Could you check a few things on this drawing? It's one solid part, dimensions in mm from its lowest x, y, z. A direction names the side the tool comes from. Coordinates: 2 decimals unless noted, no trailing zeros. Write each loop counter-clockwise with the first axis right and the second up, starting at its lowest first coordinate (ties: lowest second). Pieces come first, ordered by that corner, then holes. Notation, with made-up numbers: (73, 68) - (112, 68) arc R28 cw to (112, 90) - close; hole circle Ø10 at (46.25, -34.75). An arc over 180 degrees is marked (long way). Answer as a JSON object with one key per item and string values. Group by question number.
1) If we section it at D-D (y = 567): Write out the boundary of the cut face in (x, z).
2) We'd pull the mould along Y, two halves only. Please class the marked faces 1, 2 and 3: released by +Y, released by -Y, zero draft, split by the parting line, or undercut.
3) If we section it at A-A (y = 58.5): Write out the boundary of the cut face in (x, z).
4) On a 3-axis mill with a long thin cutter (end or side, diameter ignored), from which of +Z, -Z, +X, -X, +Y, -Y can I reach the whole of each face in a straight line? I mean the marked faces 4, 5, 6, 7 and 8. Say none if no direction works.
5) Please list where these lines run through material, in increasing order: line 1 along Y through (x, z) = (654, 82); line 2 along Y through (x, z) = (766.5, 137); line 3 along X through (y, z) = (383.5, 66).
6) If we section it at B-B (x = 444.5): State how many separate pieces and enclosed holes the cut face has, plus the area to 3 significant figures.
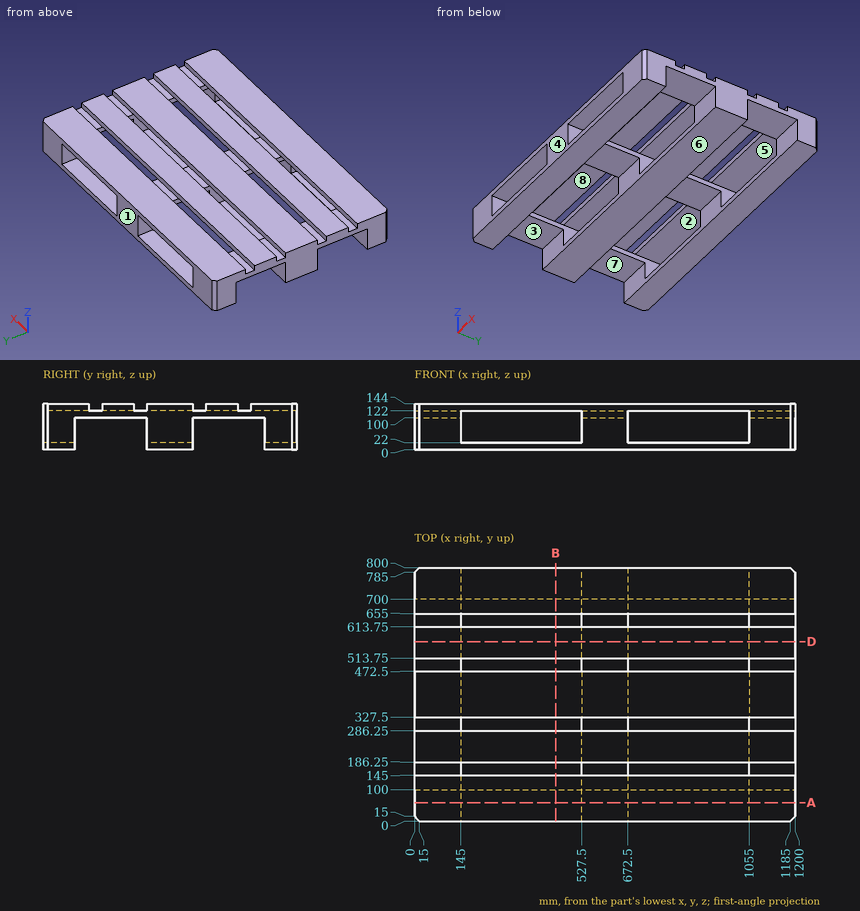
Here are the results:
{
 "1": {"outline": "(0, 100) - (145, 100) - (145, 122) - (527.5, 122) - (527.5, 100) - (672.5, 100) - (672.5, 122) - (1055, 122) - (1055, 100) - (1200, 100) - (1200, 144) - (0, 144) - close"},
 "2": {"face 1": "released by +Y", "face 2": "zero draft", "face 3": "undercut"},
 "3": {"outline": "(0, 0) - (1200, 0) - (1200, 144) - (0, 144) - close; hole (145, 22) - (527.5, 22) - (527.5, 122) - (145, 122) - close; hole (672.5, 22) - (1055, 22) - (1055, 122) - (672.5, 122) - close"},
 "4": {"face 4": "+Z, -Z, +X, -X, -Y", "face 5": "+Y, -Y", "face 6": "-Z, +X, -X, +Y, -Y", "face 7": "-Z, +X, -X", "face 8": "-Z, +Y, -Y"},
 "5": {"line 1": "y = 0 to 100, 327.5 to 472.5, 700 to 800", "line 2": "y = 0 to 145, 186.25 to 286.25, 327.5 to 472.5, 513.75 to 613.75, 655 to 800", "line 3": "x = 0 to 145, 527.5 to 672.5, 1055 to 1200"},
 "6": {"separate pieces": "8", "enclosed holes": "0", "area": "21,600 mm²"}
}
